from build123d import *

# Parameters (mm, degrees)
BASE_EXTRUDE_DEPTH                     = 254
SKETCH2_R                              = 9.9187
CUT_EXTRUDE1_DEPTH                     = 194.675
FILLET1_R                              = 6.35
SKETCH6_W                              = 190.5
SKETCH6_H                              = 66.675
CUT_EXTRUDE3_DEPTH                     = 255
FILLET2_R                              = 6.35
TAPPED_HOLE_FOR_3_4_16_HELICOIL1_D     = 19.44624
TAPPED_HOLE_FOR_3_4_16_HELICOIL1_DEPTH = 38.3032
TAPPED_HOLE_FOR_3_4_16_HELICOIL1_TIP   = 5.842239902


with BuildPart() as part:
    # Sketch1 → Base-Extrude (new body)
    with BuildSketch(Plane.XY):
        Polygon((38.494829198, 73.025), (-38.494829198, 73.025), (-78.822745501, 3.175), (-127, 3.175), (-127, 158.75), (-190.5, 158.75), (-190.5, 196.85), (190.5, 196.85), (190.5, 158.75), (127, 158.75), (127, 3.175), (78.822745501, 3.175), align=None)
    extrude(amount=BASE_EXTRUDE_DEPTH)

    # Sketch2 → Cut-Extrude1 (cut, through all)
    with BuildSketch(Plane(origin=(0, 196.85, 0), x_dir=(-1, 0, 0), z_dir=(0, 1, 0))):
        with Locations(Location((-165.1, 50.8, 0), (0, 0, 90))):  # turned: the seam where the file's is
            Circle(SKETCH2_R)
        with Locations(Location((-165.1, 203.2, 0), (0, 0, 90))):  # turned: the seam where the file's is
            Circle(SKETCH2_R)
        with Locations(Location((165.1, 203.2, 0), (0, 0, 90))):  # turned: the seam where the file's is
            Circle(SKETCH2_R)
        with Locations(Location((165.1, 50.8, 0), (0, 0, 90))):  # turned: the seam where the file's is
            Circle(SKETCH2_R)
    extrude(amount=-CUT_EXTRUDE1_DEPTH, mode=Mode.SUBTRACT)

    # Sketch5 → Cut-Revolve1 (revolve, cut)
    with BuildSketch(Plane(origin=(0, 0, 0), x_dir=(0, 0, -1), z_dir=(1, 0, 0)), mode=Mode.PRIVATE) as cut_revolve1_sk:
        with BuildLine():
            Line((-127, 171.45), (-127, 196.85))
            Line((-127, 196.85), (-16.283966834, 196.85))
            ThreePointArc((-16.283966834, 196.85), (-70.203873372, 177.881423642), (-127, 171.45))
        make_face()
    revolve(cut_revolve1_sk.sketch.rotate(Axis((0, 142.323170727, 127), (0, -1, 0)), 180), axis=Axis((0, 142.323170727, 127), (0, -1, 0)), mode=Mode.SUBTRACT)  # turned: the seam where the file's is

    # Fillet1
    fillet1_edges = [part.edges().sort_by_distance(p)[0] for p in [
        (-127, 80.9625, 0),
        (-158.75, 158.75, 0),
        (0, 196.85, 0),
        (190.5, 177.8, 0),
        (158.75, 158.75, 0),
        (127, 80.9625, 0),
        (102.911372751, 3.175, 0),
        (-102.911372751, 3.175, 0),
        (102.911372751, 3.175, 254),
        (127, 80.9625, 254),
        (-127, 3.175, 127),
        (-127, 158.75, 127),
        (-190.5, 158.75, 127),
        (-190.5, 196.85, 127),
        (190.5, 196.85, 127),
        (190.5, 158.75, 127),
        (127, 158.75, 127),
        (127, 3.175, 127),
        (158.75, 158.75, 254),
        (190.5, 177.8, 254),
        (0, 196.85, 254),
        (-190.5, 177.8, 254),
        (-158.75, 158.75, 254),
        (-127, 80.9625, 254),
        (-102.911372751, 3.175, 254),
    ]]
    fillet(fillet1_edges, radius=FILLET1_R)

    # Sketch6 → Cut-Extrude3 (cut, through all)
    with BuildSketch(Plane.XY.offset(254)):
        with Locations((0, 119.0625)):
            Rectangle(SKETCH6_W, SKETCH6_H)
    extrude(amount=-CUT_EXTRUDE3_DEPTH, mode=Mode.SUBTRACT)

    # Fillet2
    fillet2_edges = [part.edges().sort_by_distance(p)[0] for p in [
        (-95.25, 119.0625, 0),
        (-95.25, 85.725, 127),
        (0, 152.4, 254),
        (-95.25, 152.4, 127),
        (95.25, 119.0625, 0),
        (95.25, 152.4, 127),
        (0, 85.725, 254),
        (95.25, 85.725, 127),
        (0, 152.4, 0),
        (0, 85.725, 0),
        (-95.25, 119.0625, 254),
        (95.25, 119.0625, 254),
    ]]
    fillet(fillet2_edges, radius=FILLET2_R)

    # Tapped Hole for 3_4-16 Helicoil1
    with Locations(Plane.XZ.offset(-3.175)):
        with Locations((-103.124, 203.2), (-103.124, 50.8), (103.124, 203.2), (103.124, 50.8)):
            Hole(TAPPED_HOLE_FOR_3_4_16_HELICOIL1_D / 2, depth=TAPPED_HOLE_FOR_3_4_16_HELICOIL1_DEPTH)
            with Locations((0, 0, -(TAPPED_HOLE_FOR_3_4_16_HELICOIL1_DEPTH + TAPPED_HOLE_FOR_3_4_16_HELICOIL1_TIP / 2))):  # 118° drill point
                Cone(0, TAPPED_HOLE_FOR_3_4_16_HELICOIL1_D / 2, TAPPED_HOLE_FOR_3_4_16_HELICOIL1_TIP, mode=Mode.SUBTRACT)


solid = part.part
Can you work these out from the model? Positions are in its coordinate system, mm. A direction names the side the tool comes from. Round coordinates to 2 decimals unless told otherwise and drop trailing zeros. Order: outer loops, then holes, each group sorted by start corner. A loop starts at its lowest first (then second) coordinate and runs counter-clockwise, first axis right, second up. Notation, with made-up numbers: (-17.75, 50.5) -> (-13.75, 50.5) arc R27 ccw to (-13.75, 79.5) -> close; hole circle Ø9 at (-31.5, 13.5). An arc over 180 degrees is marked (long way). Write each question's results on one line, items separated by ' | '. Start each with the question number.
Item 1: If we section it at A-A, the plane y = 112.5: Write out the boundary of the cut face in (x, z).
Item 2: Thinking about a two-plate mould opening in X: for faces 4 (the flat face through (127, 82, 125)), 5 (the flat face through (-158, 158.75, 125)), 6 (the cylindrical face through (-101.016, 22.595, 193.708)), which applies, +X half, -X half, draft (parallel to the pull), parting line (faces both ways), or undercut?
Item 3: Which directions (+Z, -Z, +X, -X, +Y, -Y) give clear straight access to the entire face, cutting with the end or side of a thin tool? Please do faces 1 (the flat face through (159, 158.75, 125)), 2 (the flat face through (-58.376, 38.589, 125.222)), 3 (the cylindrical face through (-93.41, 22.59, 51.23)).
Item 4: Please list where these lines run through material, in increasing order: L1, parallel to X at y = 183, z = 203.2; L2, parallel to X at y = 29, z = 50; L3, parallel to X at y = 110.5, z = 56.5.
Item 5: If we section it at B-B, the plane x = 165.1: Write out the boundary of the cut face in (y, z), then the cut area to 3 significant figures.
Item 6: Will these pins go through, and if not, where does the flat tip stop? pin 1 (10 mm diameter, centred on x = -1.5, z = 83, fed in from +Y); pin 2 (1 mm diameter, centred on x = 13.5, z = 82.5, fed in from -Y) (3 decimals); pin 3 (16 mm diameter, centred on y = 123.5, z = 130.5, fed in from -X); pin 4 (16 mm diameter, centred on x = -165.1, z = 203.2, fed in from +Y).
Results:
1) outline: (-127, 6.35) arc R6.35 ccw to (-120.65, 0) -> (-101.6, 0) arc R6.35 ccw to (-95.25, 6.35) -> (-95.25, 247.65) arc R6.35 ccw to (-101.6, 254) -> (-120.65, 254) arc R6.35 ccw to (-127, 247.65) -> close; (95.25, 6.35) arc R6.35 ccw to (101.6, 0) -> (120.65, 0) arc R6.35 ccw to (127, 6.35) -> (127, 247.65) arc R6.35 ccw to (120.65, 254) -> (101.6, 254) arc R6.35 ccw to (95.25, 247.65) -> close
2) face 4: +X half | face 5: draft | face 6: undercut
3) face 1: +Z, -Z, +X, -Y | face 2: +Z, -Z, -Y | face 3: -Y
4) L1: x = -190.5 to -175.02, -155.18 to 155.18, 175.02 to 190.5 | L2: x = -127 to -112.81, -93.43 to -63.91, 63.91 to 93.43, 112.81 to 127 | L3: x = -127 to -95.25, 95.25 to 127
5) outline: (158.75, 6.35) arc R6.35 ccw to (165.1, 0) -> (190.5, 0) arc R6.35 ccw to (196.85, 6.35) -> (196.85, 40.88) -> (158.75, 40.88) -> close; (158.75, 60.72) -> (196.85, 60.72) -> (196.85, 193.28) -> (158.75, 193.28) -> close; (158.75, 213.12) -> (196.85, 213.12) -> (196.85, 247.65) arc R6.35 ccw to (190.5, 254) -> (165.1, 254) arc R6.35 ccw to (158.75, 247.65) -> close | area: 8,130 mm2
6) pin 1: stops at y = 176.23 | pin 2: stops at y = 73.025 | pin 3: stops at x = -127 | pin 4: passes through
